Could you check a few things on this model? Use its own coordinates, in mm. A direction names the side the tool comes from. Coordinates: 2 decimals unless noted, no trailing zeros. Order: outer loops, then holes, each group sorted by start corner. A loop starts at its lowest first (then second) coordinate and runs counter-clockwise, first axis right, second up. Notation, with made-up numbers: (60, 19.5) - (119, 19.5) arc R13 ccw to (119, 39.5) - close; hole circle Ø1 at (-1.75, 76.5). An arc over 180 degrees is marked (long way). Answer as a JSON object with one key per item and string values. Group by question number.
(1) Which directions (+Z, -Z, +X, -X, +Y, -Y) give clear straight access to the entire face, cutting with the end or side of a thin tool? Please do faces 1 (the flat face through (4, -7.55, 0)), 2 (the flat face through (2.25, -1, 0)), 3 (the flat face through (5, -5.75, 0)), 4 (the conical face through (-4.99, -5.08, 18.57)).
(2) Will these pins go through, and if not, where does the flat tip stop? P1, Ø1.2, axis at y = 1.5, z = -9.5, coming from the -X side; P2, Ø10, axis at y = -4.5, z = -12, coming from the -X side; P3, Ø6, axis at x = 3, y = 3, coming from the +Z side; P4, Ø2.5, axis at x = -4, z = 3.5, coming from the -Y side.
(3) We'd pull the mould along X, two halves only. Please class faces 5 (the cylindrical face through (-7.24, -7.4, 0.27)), 6 (the flat face through (-5.75, 5, 0)), 7 (the flat face through (-0.55, 9, 0)), 8 (the flat face through (9, -0.55, 0)): pulls with the +X half, pulls with the -X half, needs draft (parallel to the pull), parting line crosses it, or undercut.
(4) Imagine slicing it at B-B, the plane y = 1.5. Write out the boundary of the cut face in (x, z), and give its area (3 significant figures).
(5) Please list where these lines run through material, in increasing order: probe 1 along X at (y, z) = (7.75, -14); probe 2 along Y at (x, z) = (-5.5, -2); probe 3 along Y at (x, z) = (-3.75, -4).
(6) Imagine slicing it at D-D, the plane y = 5. Write out the boundary of the cut face in (x, z), and give its area (3 significant figures).
from build123d import *

# Parameters (mm, degrees)
EXTRUDE1_DEPTH     = 19
CUT_EXTRUDE1_DEPTH = 39
CUT_EXTRUDE2_DEPTH = 39


with BuildPart() as part:
    # Sketch1 → Extrude1 (new body, symmetric)
    with BuildSketch(Plane.XY):
        with BuildLine():
            Line((-10.25, 10.25), (10.25, 10.25))
            Line((10.25, 10.25), (10.25, -10.25))
            Line((10.25, -10.25), (-0.25, -10.25))
            ThreePointArc((-0.25, -10.25), (-7.321067812, -7.321067812), (-10.25, -0.25))
            Line((-10.25, -0.25), (-10.25, 10.25))
        make_face()
    extrude(amount=EXTRUDE1_DEPTH, both=True)

    # Sketch2 → Cut-Extrude1 (cut, through all)
    with BuildSketch(Plane.XY.offset(19)):
        Polygon((10.25, -7.55), (-2.75, -7.55), (-2.75, -8.75), (-0.25, -8.75), (-0.25, -10.25), (10.25, -10.25), align=None)
        Polygon((-7.55, 10.25), (-7.55, -2.75), (-8.75, -2.75), (-8.75, -0.25), (-10.25, -0.25), (-10.25, 10.25), align=None)
    extrude(amount=-CUT_EXTRUDE1_DEPTH, mode=Mode.SUBTRACT)

    # Sketch3 → Cut-Extrude2 (cut, through all)
    with BuildSketch(Plane.XY.offset(19)):
        with BuildLine():
            Line((-0.55, 10.25), (-0.55, 6.95))
            Line((-0.55, 6.95), (-2.35, 6.95))
            Line((-2.35, 6.95), (-2.35, 8.45))
            Line((-2.35, 8.45), (-5.75, 8.45))
            Line((-5.75, 8.45), (-5.75, 0.75))
            Line((-5.75, 0.75), (-2.35, 0.75))
            Line((-2.35, 0.75), (-2.35, 2.25))
            Line((-2.35, 2.25), (-0.55, 2.25))
            Line((-0.55, 2.25), (-0.55, 1.02))
            Line((-0.55, 1.02), (-3.821715344, -2.251715344))
            ThreePointArc((-3.821715344, -2.251715344), (-4.810660172, -4.810660172), (-2.251715344, -3.821715344))
            Line((-2.251715344, -3.821715344), (1.02, -0.55))
            Line((1.02, -0.55), (2.25, -0.55))
            Line((2.25, -0.55), (2.25, -2.35))
            Line((2.25, -2.35), (0.75, -2.35))
            Line((0.75, -2.35), (0.75, -5.75))
            Line((0.75, -5.75), (8.45, -5.75))
            Line((8.45, -5.75), (8.45, -2.35))
            Line((8.45, -2.35), (6.95, -2.35))
            Line((6.95, -2.35), (6.95, -0.55))
            Line((6.95, -0.55), (10.25, -0.55))
            Line((10.25, -0.55), (10.25, 10.25))
            Line((10.25, 10.25), (-0.55, 10.25))
        make_face()
    extrude(amount=-CUT_EXTRUDE2_DEPTH, mode=Mode.SUBTRACT)

    # Esboço1 → Furo roscado de M41 (revolve, cut)
    with BuildSketch(Plane(origin=(-3.75, -3.75, 19), x_dir=(0, -1, 0), z_dir=(1, 0, 0))):
        Polygon((0, 0), (0, 38), (2.25, 38), (1.65, 37.4), (1.65, 0.6), (2.25, 0), align=None)
    revolve(axis=Axis((-3.75, -3.75, 25.35), (0, 0, -1)), mode=Mode.SUBTRACT)


solid = part.part
Result set:
{
 "1": {"face 1": "+Z, -Z, +X", "face 2": "+Z, -Z, +Y", "face 3": "+Z, -Z", "face 4": "+Z"},
 "2": {"P1": "stops at x = -7.55", "P2": "stops at x = -10.25", "P3": "passes through", "P4": "stops at y = -9.93"},
 "3": {"face 5": "pulls with the -X half", "face 6": "undercut", "face 7": "pulls with the +X half", "face 8": "needs draft"},
 "4": {"outline": "(-7.55, -19) - (-5.75, -19) - (-5.75, 19) - (-7.55, 19) - close; (-2.35, -19) - (-0.55, -19) - (-0.55, 19) - (-2.35, 19) - close", "area": "137 mm^2"},
 "5": {"probe 1": "x = -7.55 to -5.75, -2.35 to -0.55", "probe 2": "y = -8.76 to 0.75, 8.45 to 10.25", "probe 3": "y = -9.62 to -5.4, -2.1 to 0.75, 8.45 to 10.25"},
 "6": {"outline": "(-7.55, -19) - (-5.75, -19) - (-5.75, 19) - (-7.55, 19) - close", "area": "68.4 mm^2"}
}
